Can you work these out from the model? Positions are in its coordinate system, mm. A direction names the side the tool comes from. Round coordinates to 2 decimals unless told otherwise and drop trailing zeros. Order: outer loops, then holes, each group sorted by start corner. A loop starts at its lowest first (then second) coordinate and runs counter-clockwise, first axis right, second up. Notation, with made-up numbers: (20.25, 52) -> (56.25, 52) arc R18 cw to (56.25, 61) -> close; hole circle Ø1 at (-38, 76). An arc over 180 degrees is marked (long way). One line per item, written item: value.
```python
from build123d import *

# Parameters (mm, degrees)
F0_R            = 40.8
F1_DEPTH        = 8
F4_R            = 3.15
F6_W            = 4.8
F6_H            = 38.4
F7_DEPTH        = 8.001
F9_DEPTH        = 8
F10_R           = 21
F11_DEPTH       = 8.001
F12_R           = 4
F14_D           = 3.3
F14_CBORE_D     = 6.5
F14_CBORE_DEPTH = 6


with BuildPart() as f1:
    # F0 (on Top) → F1 (new body)
    with BuildSketch(Plane.XY):
        Circle(F0_R)
    extrude(amount=F1_DEPTH)

    # F2 (on Right) → F3 (revolve, cut)
    with BuildSketch(Plane.YZ):
        Polygon((0, 8), (0, 0), (13.025, 0), (13.025, 6), (7.5, 6), (7.5, 8), align=None)
    revolve(axis=Axis((0, 0, 10.7360328796), (0, 0, 1)), mode=Mode.SUBTRACT)

    # F4 (on Right) → F5 (revolve, cut)
    with BuildSketch(Plane.YZ):
        with Locations((31, 9)):
            Circle(F4_R)
    revolve(axis=Axis((0, 0, 6.3867427816), (0, 0, 1)), mode=Mode.SUBTRACT)

    # F6 (on Top) → F7 (cut, through all)
    with BuildSketch(Plane.XY):
        with Locations((-38.4, 0)):
            Rectangle(F6_W, F6_H)
    extrude(amount=F7_DEPTH, mode=Mode.SUBTRACT)

    # F8 (on Top) → F9 (join, through all)
    with BuildSketch(Plane.XY):
        with BuildLine():
            Line((-45, 28.2782724184), (-45, -28.2782724184))
            Line((-45, -28.2782724184), (-12.6078933705, -38.8031058648))
            ThreePointArc((-12.6078933705, -38.8031058648), (-26.2059585661, -31.2711965814), (-36, -19.2))
            Line((-36, -19.2), (-36, 19.2))
            ThreePointArc((-36, 19.2), (-26.2059585661, 31.2711965814), (-12.6078933705, 38.8031058648))
            Line((-12.6078933705, 38.8031058648), (-45, 28.2782724184))
        make_face()
    extrude(amount=F9_DEPTH)

    # F10 (on face) → F11 (cut, through all)
    with BuildSketch(Plane.XY.offset(8)):
        with Locations((-56.25, 0)):
            Circle(F10_R)
    extrude(amount=-F11_DEPTH, mode=Mode.SUBTRACT)

    # F12
    f12_edges = [f1.edges().sort_by_distance(p)[0] for p in [
        (-45, -17.732386, 4),
        (-45, 17.732386, 4),
    ]]
    fillet(f12_edges, radius=F12_R)

    # F14 (through all)
    with Locations(Plane.XY.offset(8)):
        with Locations((-40.5, 24), (-40.5, -24), (37.5, 0)):
            CounterBoreHole(F14_D / 2, F14_CBORE_D / 2, F14_CBORE_DEPTH)


solid = f1.part
```
Q1. We'd pull the mould along Y, two halves only. Please class faces 4 (the face through (-44.6, -18.07, 4.06)), 5 (the face through (40.786, -1.077, 3.944)), 6 (the face through (-45, 24, 4)): released by +Y, released by -Y, zero draft, split by the parting line, or undercut.
Answers below:
face 4: undercut
face 5: split by the parting line
face 6: zero draft
Q2. Please list where these lines run through material, in increasing order: line 1 along Y through (x, z) = (-40.5, 1.25); line 2 along Y through (x, z) = (-1, 7); line 3 along Y through (x, z) = (18, 7.5).
Answers below:
line 1: -29.74 to -25.65, -22.35 to -13.89, 13.89 to 22.35, 25.65 to 29.74
line 2: -40.79 to -33.42, -28.55 to -7.43, 7.43 to 28.55, 33.42 to 40.79
line 3: -36.61 to -28.57, -21.75 to 21.75, 28.57 to 36.61
Q3. I want a section at A-A on x = 0. List the corners of the cut face in (y, z) for me (3 decimals).
Answers below:
outline: (-40.8, 0) -> (-13.025, 0) -> (-13.025, 6) -> (-7.5, 6) -> (-7.5, 8) -> (-28.013, 8) arc R3.15 cw to (-33.987, 8) -> (-40.8, 8) -> close; (7.5, 6) -> (13.025, 6) -> (13.025, 0) -> (40.8, 0) -> (40.8, 8) -> (33.987, 8) arc R3.15 cw to (28.013, 8) -> (7.5, 8) -> close
Q4. I want a section at B-B on y = 0. List the corners of the cut face in (x, z) for me (3 decimals), plus the area to 3 significant figures.
Answers below:
outline: (-35.25, 0) -> (-13.025, 0) -> (-13.025, 6) -> (-7.5, 6) -> (-7.5, 8) -> (-28.013, 8) arc R3.15 cw to (-33.987, 8) -> (-35.25, 8) -> close; (7.5, 6) -> (13.025, 6) -> (13.025, 0) -> (35.85, 0) -> (35.85, 2) -> (34.25, 2) -> (34.25, 8) -> (33.987, 8) arc R3.15 cw to (28.013, 8) -> (7.5, 8) -> close; (39.15, 0) -> (40.8, 0) -> (40.8, 8) -> (40.75, 8) -> (40.75, 2) -> (39.15, 2) -> close
area: 358 mm^2
Q5. On a 3-axis mill with a long thin cutter (end or side, diameter ignored), from which of +Z, -Z, +X, -X, +Y, -Y can I reach the whole of each face in a straight line? I mean faces 1 (the face through (-37.498, -25.245, 5.042)), 2 (the face through (39.15, 0.07, 0.99)), 3 (the face through (7.926, -10.336, 3.042)). Say none if no direction works.
Answers below:
face 1: +Z
face 2: +Z, -Z
face 3: -Z
Q6. I want a section at D-D on x = -40.5. List the corners of the cut face in (y, z) for me.
Answers below:
outline: (-29.74, 0) -> (-25.65, 0) -> (-25.65, 2) -> (-27.25, 2) -> (-27.25, 8) -> (-29.74, 8) -> close; (-22.35, 0) -> (-13.89, 0) -> (-13.89, 8) -> (-20.75, 8) -> (-20.75, 2) -> (-22.35, 2) -> close; (13.89, 0) -> (22.35, 0) -> (22.35, 2) -> (20.75, 2) -> (20.75, 8) -> (13.89, 8) -> close; (25.65, 0) -> (29.74, 0) -> (29.74, 8) -> (27.25, 8) -> (27.25, 2) -> (25.65, 2) -> close
Q7. I want a section at C-C on z = 1. List the corners of the cut face in (x, y) for me (3 decimals), plus the area to 3 significant figures.
Answers below:
outline: (-45, -28.278) -> (-12.608, -38.803) arc R40.8 ccw (long way) to (-12.608, 38.803) -> (-45, 28.278) -> (-45, 19.81) arc R4 ccw to (-43.44, 16.64) arc R21 cw to (-43.44, -16.64) arc R4 ccw to (-45, -19.81) -> close; hole circle Ø3.3 at (-40.5, -24); hole circle Ø3.3 at (-40.5, 24); hole circle Ø26.05 at (0, 0); hole circle Ø3.3 at (37.5, 0)
area: 5,000 mm^2
Q8. Will these pins go through, and if not, where does the flat tip stop? pin 1 Ø2 at (x, y) = (-42, -24.5) entering from +Z; pin 2 Ø1 at (x, z) = (-12, 6) entering from +Y; pin 3 Ø19.5 at (x, y) = (0, 0) entering from -Z.
Answers below:
pin 1: z = 2
pin 2: y = 39.15
pin 3: z = 6
